Can you work these out from the model? Positions are in its coordinate system, mm. Give positions to 0.01 mm unless a question says otherwise; leave off trailing zeros. Order: outer loops, then holes, each group sorted by start corner. A loop starts at its lowest first (then second) coordinate and runs counter-clockwise, first axis right, second up. Notation, with made-up numbers: M 52,-34.75 L 61,-34.75 A20 ccw 61,-11.75 Z; hole C 41,38 d5. An arc over 180 degrees is marked long. Use one line per item in the form item = value. Start each with the question number.
1. Will these pins go through, and if not, where does the flat tip stop? P1, Ø3, axis at x = 91.5, z = 15, coming from the +Y side; P2, Ø5, axis at y = 587, z = 15, coming from the -X side; P3, Ø1.5, axis at y = 243.5, z = 4, coming from the +X side.
2. I need wall thicknesses on L1, parallel to X at y = 128, z = 13.25; L2, parallel to Y at x = -37, z = 14; L3, parallel to Y at x = 121, z = 12. Which ranges of each line are inside material? Lowest first, please.
3. I want a section at B-B, the plane y = 447. List the corners of the cut face in (x, z) for me.
4. I want a section at A-A, the plane y = 142.5. List the corners of the cut face in (x, z) for me.
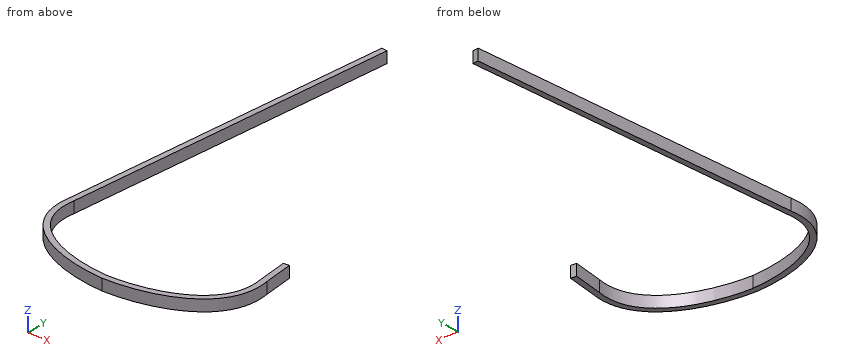
```python
from build123d import *

# Parameters (mm, degrees)
BOSS_EXTRUDE1_DEPTH = 19.05


with BuildPart() as part:
    # Sketch1 → Boss-Extrude1 (new body)
    with BuildSketch(Plane.XY):
        with BuildLine():
            Line((157.234081882, 128.980548454), (152.224173193, 179.795336584))
            Line((152.224173193, 179.795336584), (161.70321507, 180.729890008))
            Line((161.70321507, 180.729890008), (166.6875, 130.175))
            add(Edge.make_bspline(
                [(0, 0), (73.666580622, 1.740675992), (181.188092361, 36.200835609), (166.6875, 130.175)],
                knots=[0, 0, 0, 0, 1, 1, 1, 1], degree=3))
            add(Edge.make_bspline(
                [(0, 0), (-73.666580622, 1.740675992), (-181.188092361, 36.200835609), (-166.6875, 130.175)],
                knots=[0, 0, 0, 0, 1, 1, 1, 1], degree=3))
            Line((-166.6875, 130.175), (-111.860365766, 686.278790089))
            Line((-111.860365766, 686.278790089), (-102.381323889, 685.344236665))
            Line((-102.381323889, 685.344236665), (-157.234081882, 128.980548454))
            add(Edge.make_bspline(
                [(0, 9.52776174), (-1.117611602, 9.555193192), (-3.340472897, 9.624755056), (-7.880039481, 9.827207732), (-13.652210416, 10.198958437), (-20.725459036, 10.840441372), (-30.303235723, 11.962316267), (-42.47749757, 13.875858033), (-57.165232888, 17.02314898), (-71.689613059, 21.050850851), (-90.515854195, 27.626537064), (-112.436111514, 38.157452487), (-130.643933928, 51.803557723), (-142.189146149, 64.564536934), (-149.192253507, 75.075537554), (-153.541361304, 84.674022673), (-156.058613173, 92.923629982), (-157.442658539, 99.418206789), (-158.29640922, 106.242287005), (-158.540175044, 112.221426054), (-158.437150466, 117.190167219), (-158.20642164, 121.010360535), (-157.881730698, 124.277278241), (-157.584058118, 126.601085874), (-157.415798733, 127.781927866), (-157.316566229, 128.446705395), (-157.261207353, 128.804756083), (-157.234081882, 128.980548454)],
                knots=[0.001057036, 0.001057036, 0.001057036, 0.001057036, 0.016679825, 0.032302613, 0.063548191, 0.094793768, 0.126039346, 0.1885305, 0.251021655, 0.31351281, 0.376003965, 0.500986274, 0.625968584, 0.688459739, 0.750950893, 0.813442048, 0.844687626, 0.875933203, 0.90717878, 0.938424358, 0.954047147, 0.969669935, 0.985292724, 0.993104118, 0.997009815, 0.998962664, 1.000915513, 1.000915513, 1.000915513, 1.000915513], degree=3))
            add(Edge.make_bspline(
                [(157.234081882, 128.980548454), (157.261207353, 128.804756083), (157.316566229, 128.446705395), (157.415798733, 127.781927866), (157.584058118, 126.601085874), (157.881730698, 124.277278241), (158.20642164, 121.010360535), (158.437150466, 117.190167219), (158.540175044, 112.221426054), (158.29640922, 106.242287005), (157.442658539, 99.418206789), (156.058613173, 92.923629982), (153.541361304, 84.674022673), (149.192253507, 75.075537554), (142.189146149, 64.564536934), (130.643933928, 51.803557723), (112.436111514, 38.157452487), (90.515854195, 27.626537064), (71.689613059, 21.050850851), (57.165232888, 17.02314898), (42.47749757, 13.875858033), (30.303235723, 11.962316267), (20.725459036, 10.840441372), (13.652210416, 10.198958437), (7.880039481, 9.827207732), (3.340472897, 9.624755056), (1.117611602, 9.555193192), (0, 9.52776174)],
                knots=[0.001057036, 0.001057036, 0.001057036, 0.001057036, 0.003009885, 0.004962733, 0.00886843, 0.016679825, 0.032302613, 0.047925402, 0.063548191, 0.094793768, 0.126039346, 0.157284923, 0.1885305, 0.251021655, 0.31351281, 0.376003965, 0.500986274, 0.625968584, 0.688459739, 0.750950893, 0.813442048, 0.875933203, 0.90717878, 0.938424358, 0.969669935, 0.985292724, 1.000915513, 1.000915513, 1.000915513, 1.000915513], degree=3))
        make_face()
    extrude(amount=BOSS_EXTRUDE1_DEPTH)


solid = part.part
```
Check result:
q1.P1 = 29.16
q1.P2 = -121.89
q1.P3 = -145.87
q2.L1 = -167 to -157.38, 157.38 to 167
q2.L2 = 3.41 to 13.06
q2.L3 = 33.37 to 44.92
q3.outline = M -135.45,0 L -125.88,0 L -125.88,19.05 L -135.45,19.05 Z
q4.outline = M -165.47,0 L -155.9,0 L -155.9,19.05 L -165.47,19.05 Z; M 155.9,0 L 165.47,0 L 165.47,19.05 L 155.9,19.05 Z
